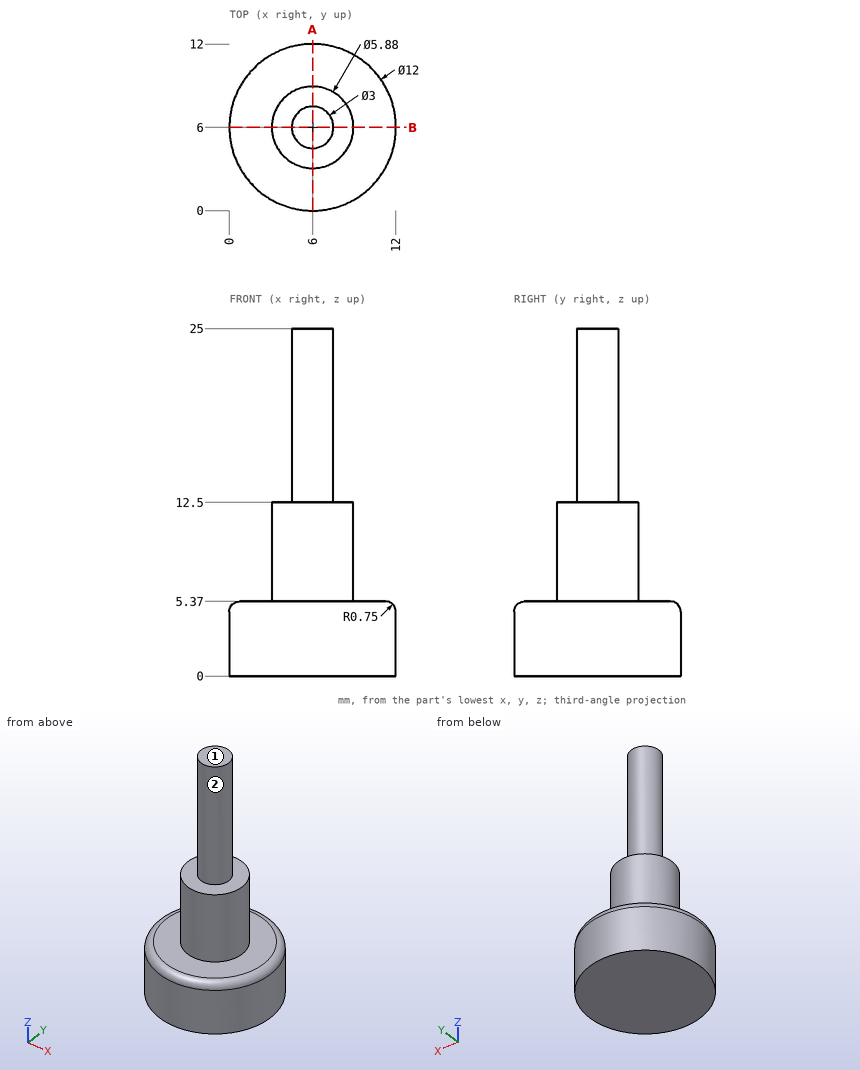
Answer from the drawing. Dimensions are ordinates in mm from the lowest x, y and z of the part. A direction names the side the tool comes from. Coordinates: 2 decimals unless noted, no trailing zeros. Loops run counter-clockwise (first coordinate to the right, second up) from the corner with the lowest first, then second, coordinate; pieces in that order, holes last.
1) Section A-A (x = 6) is taken. Give the vertices of the cut face in (y, z), plus the area to 3 significant figures.
Results:
outline: (0, 0) - (12, 0) - (12, 4.62) arc R0.75 ccw to (11.25, 5.37) - (8.94, 5.37) - (8.94, 12.5) - (7.5, 12.5) - (7.5, 25) - (4.5, 25) - (4.5, 12.5) - (3.06, 12.5) - (3.06, 5.37) - (0.75, 5.37) arc R0.75 ccw to (0, 4.62) - close
area: 144 mm2
2) Consider probe 1 along Z at (x, y) = (8.5, 5); probe 2 along Z at (x, y) = (2.5, 5.5); probe 3 along Y at (x, z) = (6, 4.75). Determine where each line is inside the solid, lowest interval first.
Results:
probe 1: z = 0 to 12.5
probe 2: z = 0 to 5.37
probe 3: y = 0.01 to 11.99
3) Flat-ended cylindrical pins translate along their axes: pin 1 (4 mm diameter, centred on x = 4.5, y = 1.5, fed in from +Z); pin 2 (1.5 mm diameter, centred on x = 9, z = 8, fed in from -Y); pin 3 (4 mm diameter, centred on x = 9, z = 21.5, fed in from -Y). Find the tip coordinate at first contact, or state that the pin passes through.
Results:
pin 1: stops at z = 12.5
pin 2: stops at y = 4.11
pin 3: stops at y = 4.88
4) For the marked faces 1 and 2, determine the directions among +Z, -Z, +X, -X, +Y, -Y from which every point of the face is accessible in a straight line to the end or side of a thin tool.
Results:
face 1: +Z, +X, -X, +Y, -Y
face 2: +Z
